```python
from build123d import *

# Parameters (mm, degrees)
F0_R       = 0.635
F1_DEPTH   = 50.8
F1_FACE_R  = 0.635
F1_FACE1_R = 0.635


with BuildPart() as f1:
    # F0 (on Top) → F1 (new body)
    with BuildSketch(Plane.XY):
        Circle(F0_R)
    extrude(amount=F1_DEPTH)

    # F3: sweep along a path in F2
    with BuildLine(Plane.XZ) as f3_path:
        ThreePointArc((7.62, 58.42), (2.2318463274, 56.1881536726), (0, 50.8))
    # F1_face (on face) → F3 (sweep)
    with BuildSketch(Plane.XY.offset(50.8)):
        Circle(F1_FACE_R)
    sweep(path=f3_path.line)

    # F5: sweep along a path in F4
    with BuildLine(Plane.XZ) as f5_path:
        ThreePointArc((0, 0), (2.2318463274, -5.3881536726), (7.62, -7.62))
    # F1_face1 (on face) → F5 (sweep)
    with BuildSketch(Plane(origin=(0, 0, 0), x_dir=(1, 0, 0), z_dir=(0, 0, -1))):
        Circle(F1_FACE1_R)
    sweep(path=f5_path.line)


solid = f1.part
```
The listing builds one solid part. Answer for the finished solid, in the listing's coordinates (mm). Round coordinates to 2 decimals unless told otherwise and drop trailing zeros. Write each loop counter-clockwise with the first axis right and the second up, starting at its lowest first coordinate (ties: lowest second). Pieces come first, ordered by that corner, then holes. Notation, with made-up numbers: (24, 88) -> (78, 88) arc R7 ccw to (78, 97) -> close; hole circle Ø7 at (12, 7.5). An arc over 180 degrees is marked (long way). Answer as a JSON object with one key per item and string values. Group by question number.
Q1. Straight lines are drawn through the part: line 1 along X through (y, z) = (-0.1, 36.5); line 2 along Z through (x, y) = (1.5, -0.2); line 3 along Z through (x, y) = (6, -0.5). For each, find the intervals that lie inside material, in ascending order.
Q2. Determine the mould class of faces 1 (the face through (-0.08, 0.63, 25.04)), 2 (the face through (7.62, 0, -8)) for opening direction Z: pulls with the +Z half, pulls with the -Z half, needs draft (parallel to the pull), parting line crosses it, or undercut.
Q3. Section B-B (z = 9.5) is taken. Write down the section's boundary in (x, y) (3 decimals), plus the area to 3 significant figures.
Q4. This flat-tipped pin is pushed along its axis until it touches: pin 1 Ø2 at (x, z) = (2, 50.5) entering from +Y. Where does it stop, or does it pass through?
Q5. Section A-A (y = 0) is taken. Write down the section's boundary in (x, z) (3 decimals), plus the area to 3 significant figures.
Check values:
{
 "1": {"line 1": "-0.63 to 0.63", "line 2": "-5.49 to -3.43, 54.23 to 56.29", "line 3": "-7.85 to -7.04, 57.84 to 58.65"},
 "2": {"face 1": "undercut", "face 2": "needs draft"},
 "3": {"outline": "circle Ø1.27 at (0, 0)", "area": "1.27 mm^2"},
 "4": {"pin 1": "through"},
 "5": {"outline": "(-0.635, 0) arc R8.255 ccw to (7.62, -8.255) -> (7.62, -6.985) arc R6.985 cw to (0.635, 0) -> (0.635, 50.8) arc R6.985 cw to (7.62, 57.785) -> (7.62, 59.055) arc R8.255 ccw to (-0.635, 50.8) -> close", "area": "94.9 mm^2"}
}
